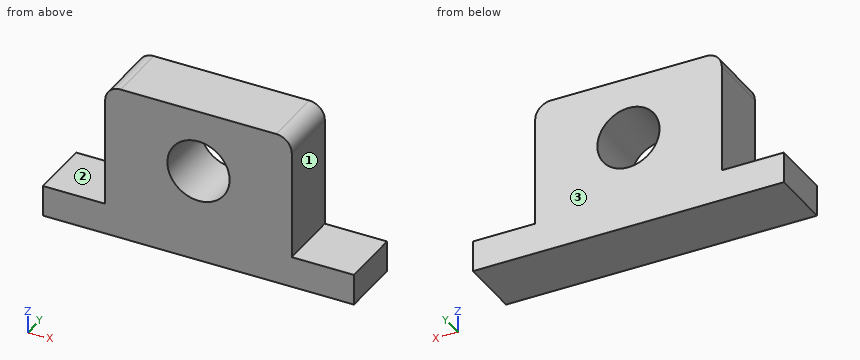
```python
from build123d import *

# Parameters (mm, degrees)
F0_R     = 12.7
F1_DEPTH = 12.7


with BuildPart() as f1:
    # F0 (on Front) → F1 (new body, symmetric)
    with BuildSketch(Plane.XZ):
        with BuildLine():
            Line((-38.1, 19.05), (-38.1, -25.4))
            Line((-38.1, -25.4), (38.1, -25.4))
            Line((38.1, -25.4), (38.1, 19.05))
            ThreePointArc((38.1, 19.05), (36.240128, 23.540128), (31.75, 25.4))
            Line((31.75, 25.4), (-31.75, 25.4))
            ThreePointArc((-31.75, 25.4), (-36.240128, 23.540128), (-38.1, 19.05))
        make_face()
        Circle(F0_R, mode=Mode.SUBTRACT)
        Polygon((-38.1, -25.4), (-63.5, -25.4), (-63.5, -38.1), (63.5, -38.1), (63.5, -25.4), (38.1, -25.4), align=None)
    extrude(amount=F1_DEPTH, both=True)


solid = f1.part
```
The listing builds one solid part. Answer for the finished solid, in the listing's coordinates (mm). Face numbers are marked on the shaded views. A direction names the side the tool comes from. Give positions to 0.01 mm unless a question says otherwise; leave off trailing zeros. Write each loop counter-clockwise with the first axis right and the second up, starting at its lowest first coordinate (ties: lowest second). Pieces come first, ordered by that corner, then holes. Notation, with made-up numbers: (39.25, -22) - (49.25, -22) arc R24 cw to (49.25, -8) - close; hole circle Ø11 at (49, 27.5). An arc over 180 degrees is marked (long way). Use one line per item in the form item = value. Start each with the question number.
1) Find section C-C on y = 5.5. Determine the outline of the cut face in (x, z), plus the area to 3 significant figures.
2) Flat-ended cylindrical pins translate along their axes: pin 1 Ø4 at (y, z) = (3, 12) entering from +X; pin 2 Ø6 at (y, z) = (1, -8.5) entering from -X; pin 3 Ø7.5 at (x, y) = (54, 0.5) entering from +Z; pin 4 Ø3 at (x, z) = (-40, -3.5) entering from -Y. Find the tip coordinate at first contact, or state that the pin passes through.
3) Consider line 1 along Z through (x, y) = (0, 2.25); line 2 along X through (y, z) = (0.75, 11); line 3 along Z through (x, y) = (-10, 7.5). Determine where each line is inside the solid, lowest interval first. Write a range as from..to.
4) Find section A-A on x = 0. Determine the outline of the cut face in (y, z), plus the area to 3 significant figures.
5) Find section B-B on z = 0. Determine the outline of the cut face in (x, y), plus the area to 3 significant figures.
6) A tool of negligible diameter and unlimited length cuts with its end or side. For the marked faces 1, 2 and 3, from which of +Z, -Z, +X, -X, +Y, -Y can it reach the whole face along a straight path? Write none if from no direction.
Geometry results:
q1.outline = (-63.5, -38.1) - (63.5, -38.1) - (63.5, -25.4) - (38.1, -25.4) - (38.1, 19.05) arc R6.35 ccw to (31.75, 25.4) - (-31.75, 25.4) arc R6.35 ccw to (-38.1, 19.05) - (-38.1, -25.4) - (-63.5, -25.4) - close; hole circle Ø25.4 at (0, 0)
q1.area = 4,960 mm2
q2.pin_1 = 38.1
q2.pin_2 = -38.1
q2.pin_3 = -25.4
q2.pin_4 = through
q3.line_1 = -38.1..-12.7, 12.7..25.4
q3.line_2 = -38.1..-6.35, 6.35..38.1
q3.line_3 = -38.1..-7.83, 7.83..25.4
q4.outline = (-12.7, -38.1) - (12.7, -38.1) - (12.7, -12.7) - (-12.7, -12.7) - close; (-12.7, 12.7) - (12.7, 12.7) - (12.7, 25.4) - (-12.7, 25.4) - close
q4.area = 968 mm2
q5.outline = (-38.1, -12.7) - (-12.7, -12.7) - (-12.7, 12.7) - (-38.1, 12.7) - close; (12.7, -12.7) - (38.1, -12.7) - (38.1, 12.7) - (12.7, 12.7) - close
q5.area = 1,290 mm2
q6.face_1 = +Z, +X, +Y, -Y
q6.face_2 = +Z, -X, +Y, -Y
q6.face_3 = +Z, -Z, +X, -X, +Y
